```python
from build123d import *

# Parameters (mm, degrees)
SKETCH1_R           = 33
SKETCH1_R_2         = 23
BOSS_EXTRUDE1_DEPTH = 26
SKETCH3_R           = 8
SKETCH3_R_2         = 1.875
BOSS_EXTRUDE2_DEPTH = 13
CUT_EXTRUDE1_DEPTH  = 5.14
BOSS_EXTRUDE3_DEPTH = 5.75
CIRPATTERN1_COUNT   = 10


with BuildPart() as part:
    # Sketch1 → Boss-Extrude1 (new body)
    with BuildSketch(Plane.XY):
        with Locations(Location((0, 0, 0), (0, 0, 180))):
            Circle(SKETCH1_R)
        with Locations(Location((0, 0, 0), (0, 0, 180))):
            Circle(SKETCH1_R_2, mode=Mode.SUBTRACT)
    extrude(amount=BOSS_EXTRUDE1_DEPTH)



with BuildPart() as body_2:
    # Sketch3 → Boss-Extrude2 (new body)
    with BuildSketch(Plane.XY):
        with Locations(Location((0, 0, 0), (0, 0, 180))):
            Circle(SKETCH3_R)
        with Locations(Location((0, 0, 0), (0, 0, 180))):
            Circle(SKETCH3_R_2, mode=Mode.SUBTRACT)
    extrude(amount=BOSS_EXTRUDE2_DEPTH)

    # Sketch4 → Cut-Extrude1 (cut)
    with BuildSketch(Plane.XY.offset(13)):
        Polygon((0, 6.92820323), (-6, 3.464101615), (-6, -3.464101615), (0, -6.92820323), (6, -3.464101615), (6, 3.464101615), align=None)
    extrude(amount=-CUT_EXTRUDE1_DEPTH, mode=Mode.SUBTRACT)


with BuildPart() as part_1:
    add(part.part)

    add(body_2.part)  # Boss-Extrude3 merges body 2
    # Sketch5 → Boss-Extrude3 (add)
    with BuildSketch(Plane.XY):
        with BuildLine():
            ThreePointArc((-1.5, 8.594163981), (-1.715299562, 8.024613517), (-2.22101797, 7.68551099))
            ThreePointArc((-2.22101797, 7.68551099), (0, 8), (2.22101797, 7.68551099))
            ThreePointArc((2.22101797, 7.68551099), (1.715299562, 8.024613517), (1.5, 8.594163981))
            Line((1.5, 8.594163981), (0.75, 22.987768487))
            ThreePointArc((0.75, 22.987768487), (0, 23), (-0.75, 22.987768487))
            Line((-0.75, 22.987768487), (-1.5, 8.594163981))
        make_face()
    boss_extrude3 = extrude(amount=BOSS_EXTRUDE3_DEPTH)

    # CirPattern1: Boss-Extrude3 ×10 about axis
    cirpattern1_axis = Axis((0, 0, 0), (0, 0, 1))
    for i in range(1, CIRPATTERN1_COUNT):
        add(boss_extrude3.rotate(cirpattern1_axis, i * 360 / CIRPATTERN1_COUNT))


solid = part_1.part
```
Build history of the part. All positions in model axes, mm. A direction names the side the tool comes from. Give positions to 0.01 mm unless a question says otherwise; leave off trailing zeros. Loops run counter-clockwise (first coordinate to the right, second up) from the corner with the lowest first, then second, coordinate; pieces in that order, holes last.
Item 1: Slice it at B-B, the plane x = 17.5. List the corners of the cut face in (y, z), and give its area (3 significant figures).
Answers follow:
outline: (-27.98, 0) - (-14.92, 0) - (-14.92, 26) - (-27.98, 26) - close; (-6.71, 0) - (-4.63, 0) - (-4.63, 5.75) - (-6.71, 5.75) - close; (4.63, 0) - (6.71, 0) - (6.71, 5.75) - (4.63, 5.75) - close; (14.92, 0) - (27.98, 0) - (27.98, 26) - (14.92, 26) - close
area: 703 mm2
Item 2: Drill centre lines: line 1 (Y direction, x = 0, z = 9); line 2 (X direction, y = -0.5, z = 12.5); line 3 (Y direction, x = -3, z = 10.25). Where is each one in solid material? Low to high.
Answers follow:
line 1: y = -33 to -23, -8 to -6.93, 6.93 to 8, 23 to 33
line 2: x = -33 to -22.99, -7.98 to -6, 6 to 7.98, 22.99 to 33
line 3: y = -32.86 to -22.8, -7.42 to -5.2, 5.2 to 7.42, 22.8 to 32.86
Item 3: Flat gauge pins, fed straight in: pin 1 (4 mm diameter, centred on x = -19, z = 17, fed in from +Y); pin 2 (12.5 mm diameter, centred on x = -7.5, y = 9.5, fed in from +Z); pin 3 (8 mm diameter, centred on x = -17, z = 18, fed in from -Y); pin 4 (3 mm diameter, centred on x = 0, y = 0, fed in from -Z). Where does each tip first touch, or does it go through?
Answers follow:
pin 1: stops at y = 28.28
pin 2: stops at z = 13
pin 3: stops at y = -30.33
pin 4: passes through
Item 4: Slice it at C-C, the plane y = -10. List the corners of the cut face in (x, z).
Answers follow:
outline: (-31.45, 0) - (-20.71, 0) - (-20.71, 26) - (-31.45, 26) - close; (-8.82, 0) - (-5.59, 0) - (-5.59, 5.75) - (-8.82, 5.75) - close; (-1.43, 0) - (1.43, 0) - (1.43, 5.75) - (-1.43, 5.75) - close; (5.59, 0) - (8.82, 0) - (8.82, 5.75) - (5.59, 5.75) - close; (20.71, 0) - (31.45, 0) - (31.45, 26) - (20.71, 26) - close
Item 5: Which spindle directions (+Z, -Z, +X, -X, +Y, -Y) get a long thin tool onto all of the face, cutting with end or side? Do faces 4 (the face through (-9, 12, 5.75)), 5 (the face through (-14.768, -5.976, 2.835)). Say none if no direction does.
Answers follow:
face 4: +Z
face 5: +Z, -Z
Item 6: Slice it at D-D, the plane z = 14.25. List the corners of the cut face in (x, y).
Answers follow:
outline: circle Ø66 at (0, 0); hole circle Ø46 at (0, 0)
Item 7: Pull direction X, two halves, no side cores. Call faces 1 (the face through (-7, 0, 0)), 2 (the face through (3, -5.4, 13)), 3 (the face through (-31.476, -9.912, 12.818)): released by +X, released by -X, zero draft, split by the parting line, or undercut.
Answers follow:
face 1: zero draft
face 2: undercut
face 3: split by the parting line
Item 8: Slice it at A-A, the plane z = 9. List the corners of the cut face in (x, y), and give its area (3 significant figures).
Answers follow:
outline: circle Ø66 at (0, 0); circle Ø16 at (0, 0); hole circle Ø46 at (0, 0); hole (-6, -3.46) - (0, -6.93) - (6, -3.46) - (6, 3.46) - (0, 6.93) - (-6, 3.46) - close
area: 1,840 mm2
